Check sheet for the drawn part. Datum: minimum x, y, z corner. Units: mm. A direction names the side the tool comes from. Give positions to 0.01 mm unless a question says otherwise; leave off trailing zeros. Order: outer loops, then holes, each group sorted by start corner. A loop starts at its lowest first (then second) coordinate and runs counter-clockwise, first axis right, second up. Notation, with made-up numbers: M 45.5,88.5 L 99.5,88.5 A31 cw 99.5,119.5 Z; hole C -34.75,-20 d8. An arc over 180 degrees is marked long. Put each result on its own line as item: value. Start each with the question number.
Q1. Go/stop test with flat-tipped pins: pin 1 (3 mm diameter, centred on x = 5, y = 14.5, fed in from -Z) (3 decimals); pin 2 (2 mm diameter, centred on y = 5.5, z = 10, fed in from -X); pin 3 (4 mm diameter, centred on x = 14, y = 9.5, fed in from +Z). Record where each tip stops, or that it passes through.
Q2. Section check D-D on z = 18.25. Record the cut outline in (x, y), then the cut area to 3 significant figures.
Q3. Material ranges on L1, parallel to Z at x = 10, y = 14.25; L2, parallel to Y at x = 5, z = 11.5; L3, parallel to Z at x = 5.25, y = 19.25, recorded low to high.
Q4. Section check B-B on y = 4. Record the cut outline in (x, z).
Q5. Section check A-A on z = 10. Record the cut outline in (x, y).
Q6. Mould release check, pull along X, two halves, no side actions. Record for the marked faces 1, 2 and 3: +X half, -X half, draft (parallel to the pull), parting line (faces both ways), or undercut.
Q7. Section check C-C on x = 16.75. Record the cut outline in (y, z) (3 decimals).
Q8. Access from +Z, -Z, +X, -X, +Y, -Y to the whole of each face (thin tool, end or side, straight path). Record for the marked faces 4, 5, 6, 7 and 8.
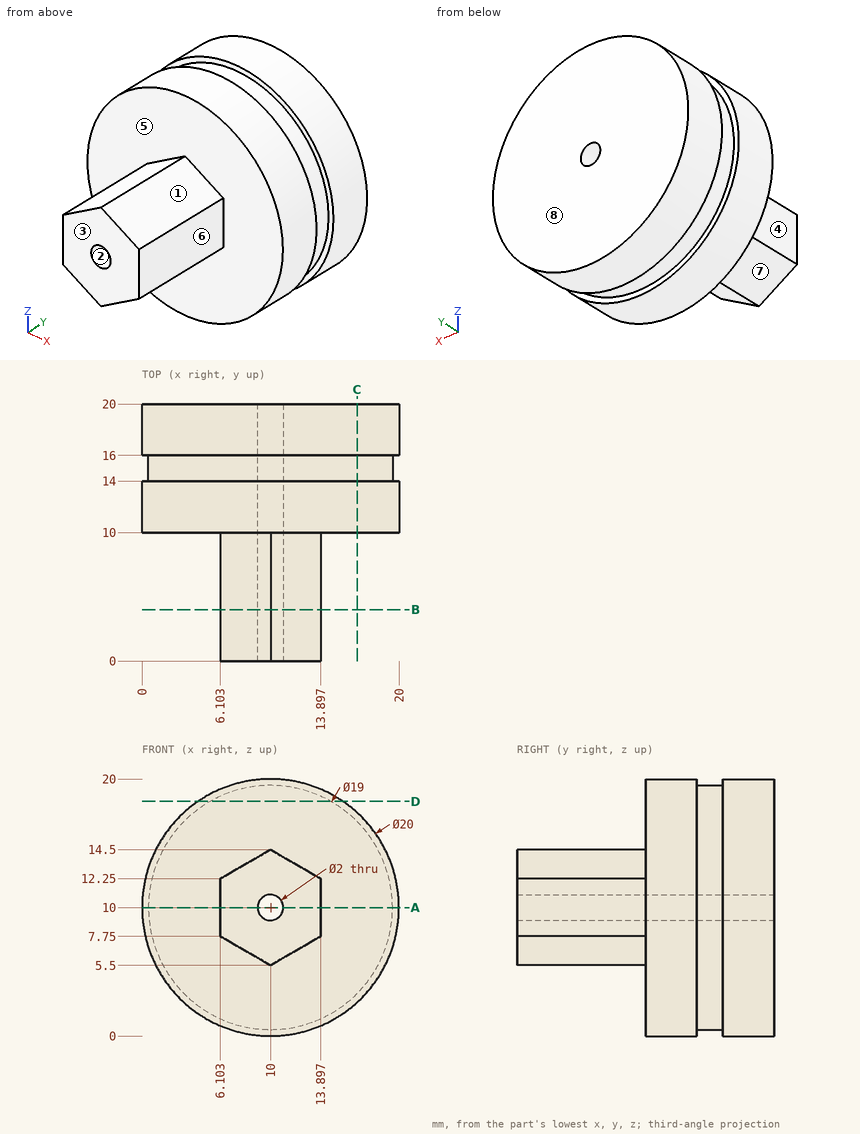
Results found:
1. pin 1: stops at z = 0.665
1. pin 2: stops at x = 6.1
1. pin 3: stops at z = 19.78
2. outline: M 4.35,10 L 15.65,10 L 15.65,14 L 14.71,14 L 14.71,16 L 15.65,16 L 15.65,20 L 4.35,20 L 4.35,16 L 5.29,16 L 5.29,14 L 4.35,14 Z
2. area: 109 mm^2
3. L1: z = 0.5 to 9, 11 to 19.5
3. L2: y = 10 to 20
3. L3: z = 1.2 to 18.8
4. outline: M 6.1,7.75 L 10,5.5 L 13.9,7.75 L 13.9,12.25 L 10,14.5 L 6.1,12.25 Z; hole C 10,10 d2
5. outline: M 0,10 L 6.1,10 L 6.1,0 L 9,0 L 9,20 L 0,20 L 0,16 L 0.5,16 L 0.5,14 L 0,14 Z; M 11,0 L 13.9,0 L 13.9,10 L 20,10 L 20,14 L 19.5,14 L 19.5,16 L 20,16 L 20,20 L 11,20 Z
6. face 1: +X half
6. face 2: undercut
6. face 3: draft
7. outline: M 10,2.622 L 14,2.622 L 14,3.315 L 16,3.315 L 16,2.622 L 20,2.622 L 20,17.378 L 16,17.378 L 16,16.685 L 14,16.685 L 14,17.378 L 10,17.378 Z
8. face 4: +Z, -Z, -X, -Y
8. face 5: -Y
8. face 6: +Z, -Z, +X, -Y
8. face 7: -Z, -X, -Y
8. face 8: +Z, -Z, +X, -X, +Y
